Verification items for the finished model (mm, model axes). A direction names the side the tool comes from. Give positions to 0.01 mm unless a question says otherwise; leave off trailing zeros. Order: outer loops, then holes, each group sorted by start corner. A loop starts at its lowest first (then second) coordinate and runs counter-clockwise, first axis right, second up.
(1) Sectioned sample at A-A on y = 6.5. Record the cut outline in (x, z).
(2) Sectioned sample at D-D on x = 19. Record the cut outline in (y, z).
(3) Mould release check, pull along Z, two halves, no side actions. Record for faces 4 (the face through (102.5, 7, 0.2)), 5 (the face through (89, 4.5, 0)), 6 (the face through (-1, -1, -12.5)): pulls with the +Z half, pulls with the -Z half, needs draft (parallel to the pull), parting line crosses it, or undercut.
(4) Sectioned sample at C-C on x = 77. Record the cut outline in (y, z).
(5) Access from +Z, -Z, +X, -X, +Y, -Y to the whole of each face (thin tool, end or side, straight path). Record for faces 1 (the face through (-89, 4.5, 0)), 2 (the face through (-102.5, 7, 0.2)), 3 (the face through (-77.5, 7, 0.2)).
(6) Scan lines: L1, parallel to X at y = 3.25, z = 0.5; L2, parallel to X at y = 6.55, z = 0; L3, parallel to Z at x = 89.5, y = 8.45. Record each from-to range of solid material in increasing order.
(7) Sectioned sample at B-B on z = 0. Record the cut outline in (x, y), plus the area to 3 significant figures.
(8) Gauge pin test, flat ends, axial feed: pin 1 (7.5 mm diameter, centred on x = -14, z = 0.5, fed in from +Y); pin 2 (8 mm diameter, centred on x = -29, y = 7, fed in from +Z); pin 3 (6 mm diameter, centred on x = 89.5, z = 0, fed in from +Y). Record the tip position at first contact, or that the pin passes through.
```python
from build123d import *

# Parameters (mm, degrees)
EXTRUDE_1_DEPTH      = 9.5
EXTRUDE_1_DEPTH_BACK = 8
SKETCH_1_W           = 210
SKETCH_1_H           = 25
SKETCH_2_W           = 150
SKETCH_2_H           = 25
CUT_EXTRUDE_1_DEPTH  = 9.5
SKETCH_3_R           = 5
CUT_EXTRUDE_2_DEPTH  = 5
CHAMFER_1_SIZE       = 5
CHAMFER_2_SIZE       = 3


with BuildPart() as part:
    # 草图1 → 凸台-拉伸1 (new, two sides: drawn at the far end of the back side and taken through both)
    with BuildSketch(Plane(origin=(0, 0, 0), x_dir=(1, 0, 0), z_dir=(0, 1, 0)).offset(-EXTRUDE_1_DEPTH_BACK)):
        Rectangle(SKETCH_1_W, SKETCH_1_H)
    extrude(amount=EXTRUDE_1_DEPTH + EXTRUDE_1_DEPTH_BACK)

    # 草图2 → 切除-拉伸1 (cut)
    with BuildSketch(Plane(origin=(0, 9.5, 0), x_dir=(1, 0, 0), z_dir=(0, 1, 0))):
        Rectangle(SKETCH_2_W, SKETCH_2_H)
    extrude(amount=-CUT_EXTRUDE_1_DEPTH, mode=Mode.SUBTRACT)

    # 草图3 → 切除-拉伸2 (cut)
    with BuildSketch(Plane(origin=(0, 9.5, 0), x_dir=(1, 0, 0), z_dir=(0, 1, 0))):
        with Locations(Location((-89.5, 0, 0), (0, 0, 270))):
            Circle(SKETCH_3_R)
        with Locations(Location((89.5, 0, 0), (0, 0, 90))):
            Circle(SKETCH_3_R)
    extrude(amount=-CUT_EXTRUDE_2_DEPTH, mode=Mode.SUBTRACT)

    # 倒角1
    chamfer_1_edges = [part.edges().sort_by_distance(p)[0] for p in [
        (-105, 9.5, 0),
        (105, 9.5, 0),
        (-75, 9.5, 0),
        (75, 9.5, 0),
    ]]
    chamfer(chamfer_1_edges, length=CHAMFER_1_SIZE)

    # 倒角2
    chamfer_2_edges = [part.edges().sort_by_distance(p)[0] for p in [
        (0, -8, -12.5),
        (0, -8, 12.5),
    ]]
    chamfer(chamfer_2_edges, length=CHAMFER_2_SIZE)


solid = part.part
```
Ans:
1. outline: (-103, -12.5) - (-77, -12.5) - (-77, 12.5) - (-103, 12.5) - close; (77, -12.5) - (103, -12.5) - (103, 12.5) - (77, 12.5) - close; hole circle Ø10 at (-89.5, 0); hole circle Ø10 at (89.5, 0)
2. outline: (-8, -9.5) - (-5, -12.5) - (0, -12.5) - (0, 12.5) - (-5, 12.5) - (-8, 9.5) - close
3. face 4: needs draft
3. face 5: undercut
3. face 6: pulls with the -Z half
4. outline: (-8, -9.5) - (-5, -12.5) - (6.5, -12.5) - (6.5, 12.5) - (-5, 12.5) - (-8, 9.5) - close
5. face 1: +Y
5. face 2: +Z, -Z, -X, +Y
5. face 3: +Z, -Z, +Y
6. L1: x = -105 to -75, 75 to 105
6. L2: x = -102.95 to -94.5, -84.5 to -77.05, 77.05 to 84.5, 94.5 to 102.95
6. L3: z = -12.5 to -5, 5 to 12.5
7. outline: (-105, -8) - (105, -8) - (105, 4.5) - (100, 9.5) - (94.5, 9.5) - (94.5, 4.5) - (84.5, 4.5) - (84.5, 9.5) - (80, 9.5) - (75, 4.5) - (75, 0) - (-75, 0) - (-75, 4.5) - (-80, 9.5) - (-84.5, 9.5) - (-84.5, 4.5) - (-94.5, 4.5) - (-94.5, 9.5) - (-100, 9.5) - (-105, 4.5) - close
7. area: 2,100 mm2
8. pin 1: stops at y = 0
8. pin 2: passes through
8. pin 3: stops at y = 4.5
